```python
from build123d import *

# Parameters (mm, degrees)
ESQUISSE1_W             = 345
ESQUISSE1_H             = 320
ESQUISSE1_R             = 4.5
ESQUISSE1_R_2           = 30
ESQUISSE1_R_3           = 35
BASE_EXTRUSION_DEPTH    = 12
ESQUISSE2_R             = 55
ESQUISSE2_R_2           = 47.5
ENL_V_MAT_EXTRU_1_DEPTH = 2
PER_AGE3_D              = 6
ESQUISSE8_R             = 9
ESQUISSE8_R_2           = 7.5
ENL_V_MAT_EXTRU_2_DEPTH = 348.230471013
ENL_V_MAT_EXTRU_3_DEPTH = 5


with BuildPart() as part:
    # Esquisse1 → Base-Extrusion (new body)
    with BuildSketch(Plane.XY):
        with Locations((32.5, -120)):
            Rectangle(ESQUISSE1_W, ESQUISSE1_H)
        with Locations((190, 25)):
            Circle(ESQUISSE1_R, mode=Mode.SUBTRACT)
        with Locations((-125, -265)):
            Circle(ESQUISSE1_R, mode=Mode.SUBTRACT)
        with Locations(Location((70, -155, 0), (0, 0, 180))):
            Circle(ESQUISSE1_R_2, mode=Mode.SUBTRACT)
        with Locations(Location((70, -30, 0), (0, 0, 180))):
            Circle(ESQUISSE1_R_3, mode=Mode.SUBTRACT)
        with Locations((-125, -70)):
            Circle(ESQUISSE1_R, mode=Mode.SUBTRACT)
    extrude(amount=BASE_EXTRUSION_DEPTH)

    # Esquisse2 → Enlèv. mat.-Extru.1 (cut)
    with BuildSketch(Plane(origin=(0, 0, 0), x_dir=(-1, 0, 0), z_dir=(0, 0, -1))):
        with Locations((-70, -30)):
            Circle(ESQUISSE2_R)
        with Locations((-70, -155)):
            Circle(ESQUISSE2_R_2)
    extrude(amount=-ENL_V_MAT_EXTRU_1_DEPTH, mode=Mode.SUBTRACT)

    # Perçage3 (through all)
    with Locations(Plane.XY.offset(12)):
        with Locations((70.60973448, 12.5), (70.358898569, -72.5), (112.5, -30), (27.5, -30), (110, -155), (70.358898569, -195), (30, -155), (70.358898569, -115)):
            Hole(PER_AGE3_D / 2)

    # Esquisse8 → Enlèv. mat.-Extru.2 (cut, through all)
    with BuildSketch(Plane.XY.offset(12)):
        with Locations((70, -262)):
            Circle(ESQUISSE8_R)
        with Locations((34, -262)):
            Circle(ESQUISSE8_R_2)
        with Locations((106, -262)):
            Circle(ESQUISSE8_R_2)
    extrude(amount=-ENL_V_MAT_EXTRU_2_DEPTH, mode=Mode.SUBTRACT)

    # Esquisse9 → Enlèv. mat.-Extru.3 (cut)
    with BuildSketch(Plane(origin=(0, 0, 0), x_dir=(-1, 0, 0), z_dir=(0, 0, -1))):
        with BuildLine():
            Line((-52, -262), (-52, -280))
            Line((-52, -280), (-88, -280))
            Line((-88, -280), (-88, -262))
            ThreePointArc((-88, -262), (-70, -244), (-52, -262))
        make_face()
    extrude(amount=-ENL_V_MAT_EXTRU_3_DEPTH, mode=Mode.SUBTRACT)


solid = part.part
```
The model under review builds one solid part; all positions refer to its coordinate system, in mm. A direction names the side the tool comes from. Round coordinates to 2 decimals unless told otherwise and drop trailing zeros. Loops run counter-clockwise (first coordinate to the right, second up) from the corner with the lowest first, then second, coordinate; pieces in that order, holes last.
Item 1: Clearance check with a flat-ended pin moving along its axis: pin 1 Ø2 at (x, z) = (85, 2) entering from -Y. State where the tip first meets the part, or that it passes through.
Determined:
pin 1: stops at y = -253.75
Item 2: Take a section at A-A (x = 190). Write out the cut boundary in (y, z).
Determined:
outline: (-280, 0) - (20.5, 0) - (20.5, 12) - (-280, 12) - close; (29.5, 0) - (40, 0) - (40, 12) - (29.5, 12) - close
Item 3: For line 1 (X direction, y = -155, z = 6.75); line 2 (Y direction, x = 110, z = 9.5); line 3 (X direction, y = -156.5, z = 7), list the stretches that pass through material, from the lowest coordinate up.
Determined:
line 1: x = -140 to 27, 33 to 40, 100 to 107, 113 to 205
line 2: y = -280 to -268.34, -255.66 to -158, -152 to -31.66, -28.34 to 40
line 3: x = -140 to 27.4, 32.6 to 40.04, 99.96 to 107.4, 112.6 to 205
Item 4: Take a section at B-B (z = 7.75). Give the number of separate pieces and of enclosed holes in the cut face, then the cut area to 3 significant figures.
Determined:
separate pieces: 1
enclosed holes: 16
area: 103,000 mm2
Item 5: Mouldability with a two-part tool opening along X and no side actions: class faces 4 (the face through (-128.6, -267.7, 5.9)), 5 (the face through (-140, -122, 6)), 6 (the face through (30, -118, 0)) as released by +X, released by -X, zero draft, split by the parting line, or undercut.
Determined:
face 4: undercut
face 5: released by -X
face 6: zero draft
Item 6: For faces 1 (the face through (109.461, -268.654, 6.084)), 2 (the face through (70, -244, 2)), 3 (the face through (114, -63, 1)), list the 3-axis set-ups (+Z, -Z, +X, -X, +Y, -Y) from which the entire face can be reached by the end or side of a thin tool; tool diameter is ignored.
Determined:
face 1: +Z, -Z
face 2: -Z, -Y
face 3: -Z
